The drawing under review shows one solid part. Ordinate dimensions are in mm from its lowest x, y, z. A direction names the side the tool comes from. Coordinates: 2 decimals unless noted, no trailing zeros. Order: outer loops, then holes, each group sorted by start corner. A loop starts at its lowest first (then second) coordinate and runs counter-clockwise, first axis right, second up.
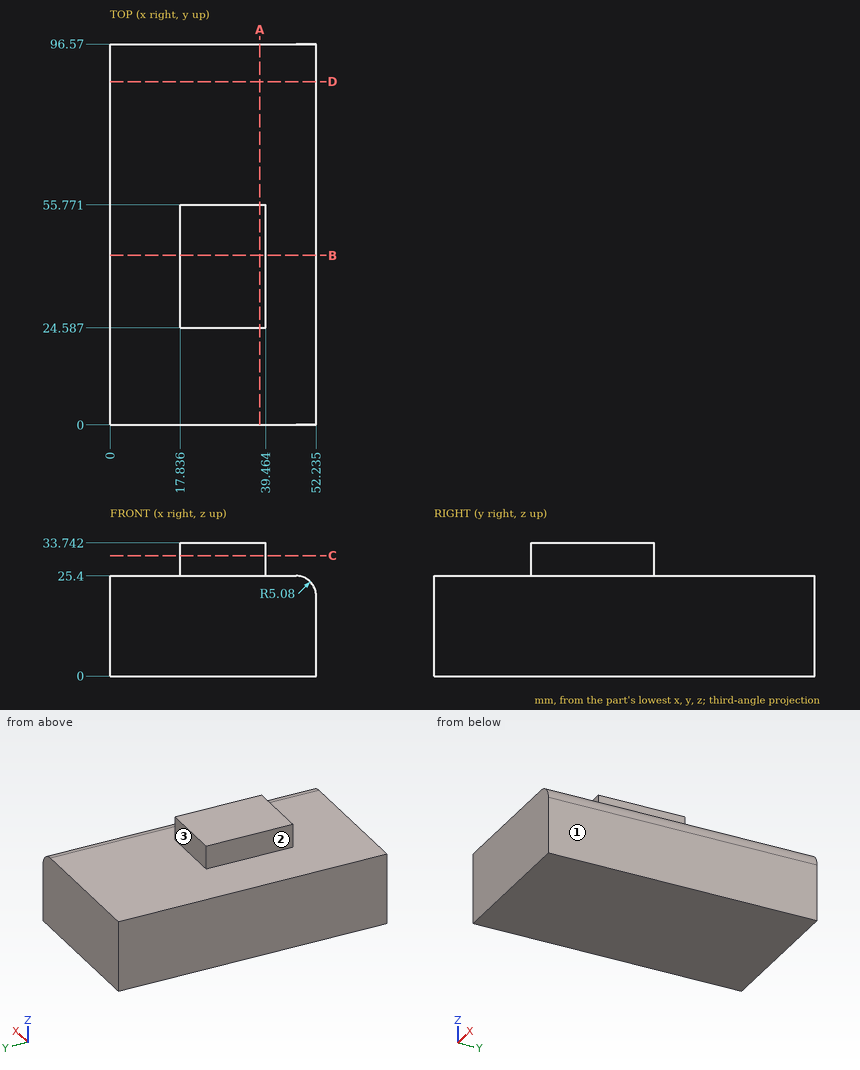
1. Add section D-D (y = 87). Give the boundary of the cut face in (x, z) (1 decimal), and give its area (3 significant figures).
2. Add section B-B (y = 43). Give the boundary of the cut face in (x, z) (1 decimal), and give its area (3 significant figures).
3. To check wall thickness, follow line 1 (Z direction, x = 47, y = 10.5); line 2 (X direction, y = 52, z = 23); line 3 (X direction, y = 82.5, z = 25) (1 decimal). State the ranges of each line that lie inside material, in increasing order.
4. Insertion check: pin 1 (2.5 mm diameter, centred on y = 47.5, z = 31, fed in from +X); pin 2 (2 mm diameter, centred on x = 9, y = 45.5, fed in from +Z); pin 3 (6.5 mm diameter, centred on y = 39.5, z = 29, fed in from -X). Each pin has a flat end and moves straight along its axis. Give the tip position at first contact, or say it passes through.
5. For the marked faces 1, 2 and 3, list the 3-axis set-ups (+Z, -Z, +X, -X, +Y, -Y) from which the entire face can be reached by the end or side of a thin tool; tool diameter is ignored.
6. Add section A-A (x = 38). Give the boundary of the cut face in (y, z).
7. Add section C-C (z = 30.5). Give the boundary of the cut face in (x, y) (1 decimal).
Solution:
1. outline: (0, 0) - (52.2, 0) - (52.2, 20.3) arc R5.1 ccw to (47.2, 25.4) - (0, 25.4) - close
1. area: 1,320 mm2
2. outline: (0, 0) - (52.2, 0) - (52.2, 20.3) arc R5.1 ccw to (47.2, 25.4) - (39.5, 25.4) - (39.5, 33.7) - (17.8, 33.7) - (17.8, 25.4) - (0, 25.4) - close
2. area: 1,500 mm2
3. line 1: z = 0 to 25.4
3. line 2: x = 0 to 51.47
3. line 3: x = 0 to 49.1
4. pin 1: stops at x = 39.46
4. pin 2: stops at z = 25.4
4. pin 3: stops at x = 17.84
5. face 1: +Z, -Z, +X, +Y, -Y
5. face 2: +Z, -X, +Y, -Y
5. face 3: +Z, +X, -X, +Y
6. outline: (0, 0) - (96.57, 0) - (96.57, 25.4) - (55.77, 25.4) - (55.77, 33.74) - (24.59, 33.74) - (24.59, 25.4) - (0, 25.4) - close
7. outline: (17.8, 24.6) - (39.5, 24.6) - (39.5, 55.8) - (17.8, 55.8) - close
